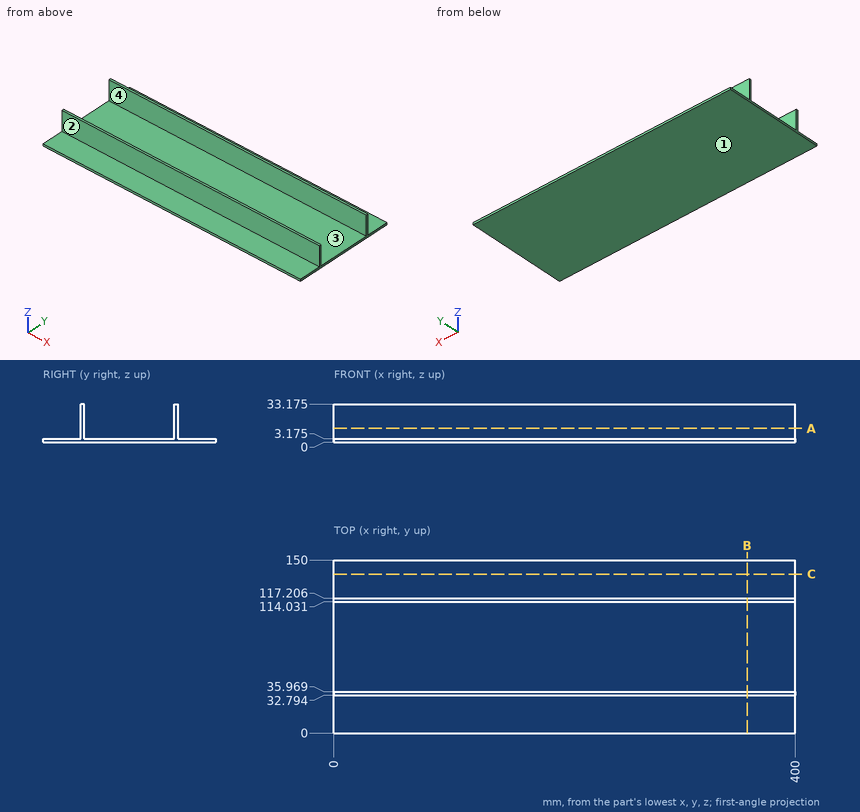
Source: three-view drawing plus pictorial views. Frame: mm from the lowest corner of the part. Give positions to 0.01 mm unless a question says otherwise; leave off trailing zeros. Write each loop counter-clockwise with the first axis right and the second up, starting at its lowest first coordinate (ties: lowest second). Pieces come first, ordered by that corner, then holes. Notation, with made-up numbers: (77, 44.25) -> (88, 44.25) arc R25 ccw to (88, 79.25) -> close; hole circle Ø3 at (11.25, 12.25). An arc over 180 degrees is marked (long way). Answer in a Markdown table with one row per item.
(1) Draft query along Y for the marked faces 1, 2, 3 and 4. Return one class per face: +Y half, -Y half, draft (parallel to the pull), parting line (faces both ways), or undercut.
Answers below:
| item | result |
|---|---|
| face 1 | draft |
| face 2 | -Y half |
| face 3 | undercut |
| face 4 | undercut |
(2) Ray query, line 1 along Y through (x, z) = (248, 7) (1 decimal); line 2 along Z through (x, y) = (152.5, 110) (1 decimal). Return the intervals inside material, ascending. Write a range as [from, to].
Answers below:
| item | result |
|---|---|
| line 1 | [32.8, 36], [114, 117.2] |
| line 2 | [0, 3.2] |
(3) Pin query (flat end, axial travel): pin 1 (2 mm diameter, centred on x = 225.5, z = 30, fed in from -Y); pin 2 (16.5 mm diameter, centred on x = 266, y = 20, fed in from +Z) (3 decimals); pin 3 (10 mm diameter, centred on x = 152, z = 12, fed in from +Y). Return the tip coordinate at first contact, or that it passes through.
Answers below:
| item | result |
|---|---|
| pin 1 | y = 32.79 |
| pin 2 | z = 3.175 |
| pin 3 | y = 117.21 |
(4) Section query A-A on z = 12. Return loops of the section in (x, y) (1 decimal).
Answers below:
| item | result |
|---|---|
| outline | (0, 32.8) -> (400, 32.8) -> (400, 36) -> (0, 36) -> close; (0, 114) -> (400, 114) -> (400, 117.2) -> (0, 117.2) -> close |
(5) Section query C-C on y = 138. Return loops of the section in (x, z) (1 decimal), then the cut area to 3 significant figures.
Answers below:
| item | result |
|---|---|
| outline | (0, 0) -> (400, 0) -> (400, 3.2) -> (0, 3.2) -> close |
| area | 1,270 mm^2 |
(6) Section query B-B on x = 358.5. Return loops of the section in (y, z) (1 decimal).
Answers below:
| item | result |
|---|---|
| outline | (0, 0) -> (150, 0) -> (150, 3.2) -> (117.2, 3.2) -> (117.2, 33.2) -> (114, 33.2) -> (114, 3.2) -> (36, 3.2) -> (36, 33.2) -> (32.8, 33.2) -> (32.8, 3.2) -> (0, 3.2) -> close |
